Could you check a few things on this model? Use its own coordinates, in mm. A direction names the side the tool comes from. Give positions to 0.01 mm unless a question says otherwise; leave off trailing zeros. Order: outer loops, then holes, each group sorted by start corner. A loop starts at its lowest first (then second) coordinate and runs counter-clockwise, first axis right, second up. Notation, with made-up numbers: (12.5, 82) -> (71.5, 82) arc R25 cw to (71.5, 96) -> close; hole circle Ø3 at (0.5, 54). An arc over 180 degrees is marked (long way). One line per item, written item: value.
```python
from build123d import *

# Parameters (mm, degrees)
F0_R     = 9.525
F0_R_2   = 1.5875
F1_DEPTH = 50.8
F2_R     = 6.35
F3_DEPTH = 25.4
F4_R     = 3.175
F5_DEPTH = 9.526


with BuildPart() as f1:
    # F0 (on Top) → F1 (new body)
    with BuildSketch(Plane.XY):
        Circle(F0_R)
        Circle(F0_R_2, mode=Mode.SUBTRACT)
    extrude(amount=F1_DEPTH)

    # F2 (on face) → F3 (cut)
    with BuildSketch(Plane.XY.offset(50.8)):
        Circle(F2_R)
    extrude(amount=-F3_DEPTH, mode=Mode.SUBTRACT)

    # F4 (on Right) → F5 (cut, through all)
    with BuildSketch(Plane.YZ):
        with Locations((0, 12.7)):
            Circle(F4_R)
        with Locations((0, 38.1)):
            Circle(F4_R)
    extrude(amount=-F5_DEPTH, mode=Mode.SUBTRACT)


solid = f1.part
```
1) Suppose I cut it at A-A, the plane y = 0. State how many separate pieces and enclosed holes the cut face has, then the cut area to 3 significant figures.
Answer below:
separate pieces: 4
enclosed holes: 0
area: 494 mm2
2) Suppose I cut it at B-B, the plane x = -1. Write out the boundary of the cut face in (y, z) (3 decimals), then the cut area to 3 significant figures.
Answer below:
outline: (-9.472, 0) -> (-1.233, 0) -> (-1.233, 9.774) arc R3.175 cw to (-1.233, 15.626) -> (-1.233, 25.4) -> (-6.271, 25.4) -> (-6.271, 50.8) -> (-9.472, 50.8) -> close; (1.233, 0) -> (9.472, 0) -> (9.472, 50.8) -> (6.271, 50.8) -> (6.271, 25.4) -> (1.233, 25.4) -> (1.233, 15.626) arc R3.175 cw to (1.233, 9.774) -> close
area: 565 mm2
3) For faces 5 (the cylindrical face through (6.057, 1.907, 38.278)), 6 (the flat face through (2, 0, 0)), 7 (the cylindrical face through (-7.49, 3.03, 39.05)), which set-ups out of +Z, -Z, +X, -X, +Y, -Y let a thin tool reach every point of the face, with its end or its side?
Answer below:
face 5: +Z
face 6: -Z, +X, -X, +Y, -Y
face 7: -X
4) Suppose I cut it at D-D, the plane x = -4.5. Write out the boundary of the cut face in (y, z) (3 decimals).
Answer below:
outline: (-8.395, 0) -> (8.395, 0) -> (8.395, 50.8) -> (4.48, 50.8) -> (4.48, 25.4) -> (-4.48, 25.4) -> (-4.48, 50.8) -> (-8.395, 50.8) -> close; hole circle Ø6.35 at (0, 12.7)
5) For P1, Ø1.3, axis at y = 3, z = 12, coming from the -X side; P2, Ø3, axis at y = 4, z = 34.5, coming from the +X side; P3, Ø1.5, axis at y = -7, z = 40, coming from the +X side, each with a flat end and sliding along its axis, tell me the tip position at first contact or that it passes through.
Answer below:
P1: stops at x = -9.08
P2: stops at x = 9.19
P3: stops at x = 7.19
6) If I drill on line 1 along Z through (x, y) = (-7, 1); line 2 along Y through (x, z) = (0, 36.25) (3 decimals); line 3 along Y through (x, z) = (0, 6.75) (1 decimal), over which ranges is the centre line in solid material (lowest first)?
Answer below:
line 1: z = 0 to 9.69, 15.71 to 35.09, 41.11 to 50.8
line 2: y = -9.525 to -6.35, 6.35 to 9.525
line 3: y = -9.5 to -1.6, 1.6 to 9.5
7) We'd pull the mould along Y, two halves only. Please class faces 1 (the cylindrical face through (9.085, 2.861, 25.044)), 2 (the flat face through (2, -6.2, 50.8)), 3 (the flat face through (0, -2, 13)), 4 (the cylindrical face through (1.514, 0.477, 12.522)): +Y half, -Y half, draft (parallel to the pull), parting line (faces both ways), or undercut.
Answer below:
face 1: parting line
face 2: draft
face 3: undercut
face 4: undercut
